from build123d import *

# Parameters (mm, degrees)
SKETCH1_R               = 2.5
BOSS_EXTRUDE1_DEPTH     = 28.879
SKETCH2_R               = 2.5
CUT_EXTRUDE1_DEPTH      = 5
CUT_EXTRUDE2_DEPTH      = 13.1
CUT_EXTRUDE3_DEPTH      = 3.5
CUT_EXTRUDE3_DEPTH_BACK = 3.5


with BuildPart() as part:
    # Sketch1 → Boss-Extrude1 (new body)
    with BuildSketch(Plane.XY):
        Circle(SKETCH1_R)
    extrude(amount=BOSS_EXTRUDE1_DEPTH)

    # Sketch2 → Cut-Extrude1 (cut)
    with BuildSketch(Plane(origin=(0, 0, 0), x_dir=(-1, 0, 0), z_dir=(0, 0, -1))):
        Circle(SKETCH2_R)
        with BuildLine():
            Line((-1.5, 1.322875656), (-1.5, -1.322875656))
            ThreePointArc((-1.5, -1.322875656), (0, -2), (1.5, -1.322875656))
            Line((1.5, -1.322875656), (1.5, 1.322875656))
            ThreePointArc((1.5, 1.322875656), (0, 2), (-1.5, 1.322875656))
        make_face(mode=Mode.SUBTRACT)
    extrude(amount=-CUT_EXTRUDE1_DEPTH, mode=Mode.SUBTRACT)

    # Sketch3 → Cut-Extrude2 (cut)
    with BuildSketch(Plane.XY.offset(28.879)):
        with BuildLine():
            Line((-1.5, 2), (1.5, 2))
            ThreePointArc((1.5, 2), (0, 2.5), (-1.5, 2))
        make_face()
        with BuildLine():
            Line((-1.5, -2), (1.5, -2))
            ThreePointArc((1.5, -2), (0, -2.5), (-1.5, -2))
        make_face()
    extrude(amount=-CUT_EXTRUDE2_DEPTH, mode=Mode.SUBTRACT)

    # Sketch4 → Cut-Extrude3 (cut, two sides)
    with BuildSketch(Plane(origin=(0, 0, 0), x_dir=(0, 0, -1), z_dir=(1, 0, 0))) as cut_extrude3_sk:
        with BuildLine():
            Line((-15.779, 2.5), (-15.779, 2))
            ThreePointArc((-15.779, 2), (-15.425446609, 2.146446609), (-15.279, 2.5))
            Line((-15.279, 2.5), (-15.779, 2.5))
        make_face()
        with BuildLine():
            Line((-15.779, -2.5), (-15.779, -2))
            ThreePointArc((-15.779, -2), (-15.425446609, -2.146446609), (-15.279, -2.5))
            Line((-15.279, -2.5), (-15.779, -2.5))
        make_face()
    extrude(amount=CUT_EXTRUDE3_DEPTH, mode=Mode.SUBTRACT)
    extrude(cut_extrude3_sk.sketch, amount=-CUT_EXTRUDE3_DEPTH_BACK, mode=Mode.SUBTRACT)


solid = part.part
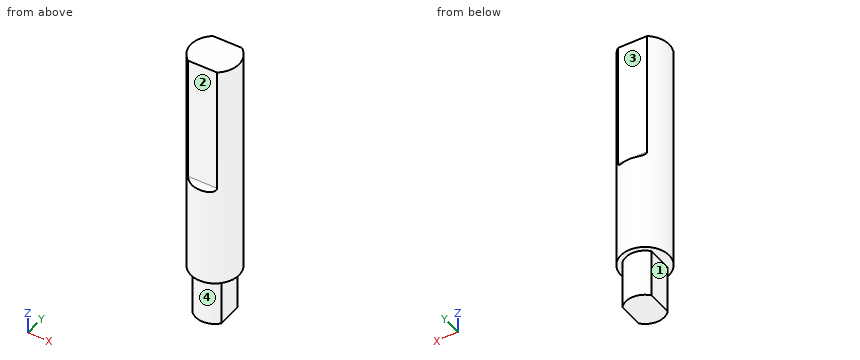
Source: CAD feature listing. Evaluate the final solid. Frame: model axes, mm. Face numbers are marked on the shaded views. A direction names the side the tool comes from. Coordinates: 2 decimals unless noted, no trailing zeros. Loops run counter-clockwise (first coordinate to the right, second up) from the corner with the lowest first, then second, coordinate; pieces in that order, holes last. Notation, with made-up numbers: M 18,82 L 38,82 A24 cw 38,98 Z; hole C -29.5,24 d6. An arc over 180 degrees is marked long. Answer in a Markdown table with one row per item.
Q1. Set-up query: the marked faces 1, 2, 3 and 4. Return all of +Z, -Z, +X, -X, +Y, -Y with unobstructed straight access to the full face (end or side cutting, diameter ignored); none if empty.
Answers below:
| item | result |
|---|---|
| face 1 | -Z, -X, +Y, -Y |
| face 2 | +Z, +X, -X, -Y |
| face 3 | +Z, +X, -X, +Y |
| face 4 | -Z, -Y |
Q2. Section D-D on z = 26.5. Return the cut outline in (x, y), plus the area to 3 significant figures.
Answers below:
| item | result |
|---|---|
| outline | M -1.5,-2 L 1.5,-2 A2.5 ccw 1.5,2 L -1.5,2 A2.5 ccw Z |
| area | 17.6 mm^2 |
Q3. Section C-C on z = 12.5. Return the cut outline in (x, y), plus the area to 3 significant figures.
Answers below:
| item | result |
|---|---|
| outline | C 0,0 d5 |
| area | 19.6 mm^2 |
Q4. First-contact query: pin 1 (0.8 mm diameter, centred on y = 0.5, z = 2.5, fed in from +X); pin 2 (2.5 mm diameter, centred on x = 0, z = 23.5, fed in from -Y); pin 3 (1.3 mm diameter, centred on y = 0, z = 2, fed in from -X). Flat tips, straight axial feed; report the tip coordinate or a pass-through.
Answers below:
| item | result |
|---|---|
| pin 1 | stops at x = 1.5 |
| pin 2 | stops at y = -2 |
| pin 3 | stops at x = -1.5 |
Q5. Ray query, probe 1 along Y at (x, z) = (1.35, 26.5); probe 2 along Z at (x, y) = (-1.75, -0.95). Return the intervals inside material, ascending. Write a range as from..to.
Answers below:
| item | result |
|---|---|
| probe 1 | y = -2..2 |
| probe 2 | z = 5..28.88 |
Q6. Section A-A on y = 0. Return the cut outline in (x, z).
Answers below:
| item | result |
|---|---|
| outline | M -2.5,5 L -1.5,5 L -1.5,0 L 1.5,0 L 1.5,5 L 2.5,5 L 2.5,28.88 L -2.5,28.88 Z |
Q7. Section B-B on x = 0. Return the cut outline in (y, z).
Answers below:
| item | result |
|---|---|
| outline | M -2.5,5 L -2,5 L -2,0 L 2,0 L 2,5 L 2.5,5 L 2.5,15.28 A0.5 cw 2,15.78 L 2,28.88 L -2,28.88 L -2,15.78 A0.5 cw -2.5,15.28 Z |
